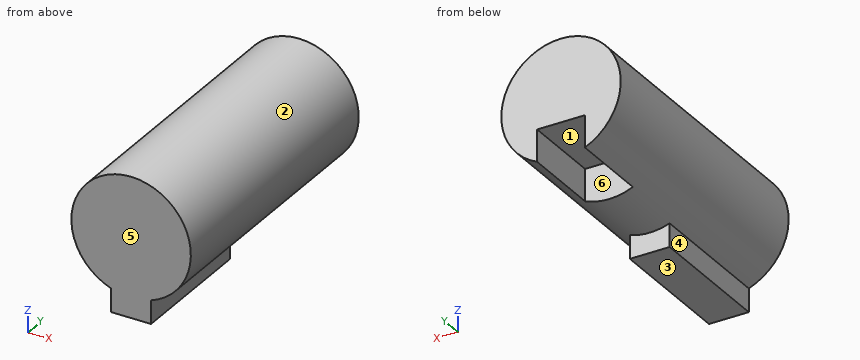
```python
from build123d import *

# Parameters (mm, degrees)
SKETCH_1_R          = 3
EXTRUDE_2_DEPTH     = 14
EXTRUDE_3_DEPTH     = 6.6
CUT_EXTRUDE_1_DEPTH = 4


with BuildPart() as part:
    # Sketch 1 → Extrude 2 (new body)
    with BuildSketch(Plane(origin=(0, 0, 0), x_dir=(1, 0, 0), z_dir=(0, 1, 0))):
        with Locations(Location((0, 0, 0), (0, 0, 270))):
            Circle(SKETCH_1_R)
    extrude(amount=EXTRUDE_2_DEPTH)

    # Sketch 1_3 → Extrude 3 (add)
    with BuildSketch(Plane(origin=(0, 0, 0), x_dir=(1, 0, 0), z_dir=(0, 1, 0))):
        with BuildLine():
            Line((-1, 4), (-1, 2.828427125))
            ThreePointArc((-1, 2.828427125), (0, 3), (1, 2.828427125))
            Line((1, 2.828427125), (1, 4))
            Line((1, 4), (-1, 4))
        make_face()
    extrude(amount=EXTRUDE_3_DEPTH)

    # Sketch 2 → Cut-Extrude 1 (cut)
    with BuildSketch(Plane(origin=(0, 14, 0), x_dir=(1, 0, 0), z_dir=(0, 1, 0))):
        Polygon((-1.2, 1.149545417), (1.2, 1.149545417), (1.2, 2.749545417), (0, 4.828006386), (-1.2, 2.749545417), align=None)
    extrude(amount=-CUT_EXTRUDE_1_DEPTH, mode=Mode.SUBTRACT)


solid = part.part
```
CAD build for the part. Positions are in the model's coordinates, mm. Face numbers are marked on the shaded views. A direction names the side the tool comes from. Coordinates: 2 decimals unless noted, no trailing zeros. Order: outer loops, then holes, each group sorted by start corner. A loop starts at its lowest first (then second) coordinate and runs counter-clockwise, first axis right, second up. Notation, with made-up numbers: M 2.25,38 L 55.25,38 A28 cw 55.25,59 Z; hole C 43.25,66 d8. An arc over 180 degrees is marked long. Answer as CSV lines item,"result".
1) Cut at D-D (y = 7.5). List the corners of the cut face in (x, z).
Verdict:
outline,"C 0,0 d6"
2) Flat gauge pins, fed straight in: P1, Ø0.5, axis at y = 12.5, z = -2.5, coming from the -X side; P2, Ø1.8, axis at y = 11, z = -2, coming from the +X side; P3, Ø3, axis at y = 1.5, z = -3.5, coming from the -X side. Where does each tip first touch, or does it go through?
Verdict:
P1,"x = -1.98"
P2,"x = 2.79"
P3,"x = -2.24"
3) Mould opens along X. For the marked faces 1, 2, 3 and 4 say: released by +X, released by -X, zero draft, split by the parting line, or undercut.
Verdict:
face 1,"undercut"
face 2,"split by the parting line"
face 3,"zero draft"
face 4,"released by -X"
4) Cut at B-B (y = 13.25). List the corners of the cut face in (x, z).
Verdict:
outline,"M -1.2,-2.75 L -1.2,-1.15 L 1.2,-1.15 L 1.2,-2.75 A3 ccw long Z"
5) 3-axis set-ups, long thin cutter, end or side, ignore diameter. For the marked faces 5 and 6: which of +Z, -Z, +X, -X, +Y, -Y reach the whole face in a straight line?
Verdict:
face 5,"+Z, -Z, +X, -X, -Y"
face 6,"-Z, +Y"
6) Cut at C-C (z = -2). List the corners of the cut face in (x, y), then the cut area to 3 significant figures.
Verdict:
outline,"M -2.24,0 L 2.24,0 L 2.24,14 L 1.2,14 L 1.2,10 L -1.2,10 L -1.2,14 L -2.24,14 Z"
area,"53.0 mm2"
7) Cut at A-A (x = 0). List the corners of the cut face in (y, z).
Verdict:
outline,"M 0,-4 L 6.6,-4 L 6.6,-3 L 10,-3 L 10,-1.15 L 14,-1.15 L 14,3 L 0,3 Z"
8) Drill centre lines: L1, parallel to Y at x = 0.5, z = -1.75; L2, parallel to Y at x = 0.65, z = -3; L3, parallel to X at y = 10.5, z = -1.5. Where is each one in solid material? Low to high. Write a range as from..to.
Verdict:
L1,"0..10"
L2,"0..6.6"
L3,"-2.6..-1.2, 1.2..2.6"
